from build123d import *

# Parameters (mm, degrees)
PAD_DEPTH            = 6.5
POCKET_DEPTH         = 6
SKETCH002_R          = 13.5
POCKET001_DEPTH      = 1
SKETCH003_W          = 6.45
SKETCH003_H          = 6.5
PAD001_DEPTH         = 3.5
POCKET002_DEPTH      = 10
SKETCH010_W          = 5
SKETCH010_H          = 6.5
PAD002_DEPTH         = 3.5
POCKET005_DEPTH      = 10
SKETCH015_R          = 2.2
SKETCH015_R_2        = 1.025
PAD003_DEPTH         = 2
POCKET009_DEPTH      = 4
POCKET010_DEPTH      = 4
PAD004_DEPTH         = 4
POCKET013_DEPTH      = 13.201
POCKET013_DEPTH_BACK = 35.201
SKETCH022_R          = 0.6
POCKET014_DEPTH      = 2
SKETCH023_R          = 0.6
POCKET015_DEPTH      = 2
SKETCH024_R          = 13.5
PAD005_DEPTH         = 0.5
SKETCH025_R          = 20.45
SKETCH025_R_2        = 19.85
POCKET016_DEPTH      = 0.3
SKETCH026_R          = 1
POCKET017_DEPTH      = 5


with BuildPart() as part:
    # Sketch → Pad (new body)
    with BuildSketch(Plane.XY):
        with BuildLine():
            Line((-22.5019915649, 16), (-22.5019915649, -16))
            Line((-22.5019915649, -16), (-16.2858834578, -17.9))
            ThreePointArc((-16.2858834578, -17.9), (-0.4552796053, -24.1957169863), (15.6009615088, -18.5))
            Line((15.6009615088, -18.5), (24.5395016581, -17.45))
            Line((24.5395016581, 17.45), (24.5395016581, -17.45))
            Line((15.6009615088, 18.5), (24.5395016581, 17.45))
            ThreePointArc((15.6009615088, 18.5), (-0.4552796053, 24.1957169863), (-16.2858834578, 17.9))
            Line((-22.5019915649, 16), (-16.2858834578, 17.9))
        make_face()
    extrude(amount=PAD_DEPTH)

    # Sketch001 → Pocket (cut)
    with BuildSketch(Plane.XY):
        with BuildLine():
            Line((-14.8539557021, 16.9), (-21.2122180433, 15.55))
            Line((-21.2122180433, 15.55), (-21.2122180433, -15.55))
            Line((-21.2122180433, -15.55), (-14.8539557021, -16.9))
            ThreePointArc((-14.8539557021, -16.9), (-0.0760301383, -22.4998715423), (14.739402973, -17))
            Line((14.739402973, -17), (23.6191552218, -16.4))
            Line((23.6191552218, 16.4), (23.6191552218, -16.4))
            Line((14.739402973, 17), (23.6191552218, 16.4))
            ThreePointArc((14.739402973, 17), (-0.0760301383, 22.4998715423), (-14.8539557021, 16.9))
        make_face()
    extrude(amount=POCKET_DEPTH, mode=Mode.SUBTRACT)

    # Sketch002 (on Face19 of Pocket) → Pocket001 (cut)
    with BuildSketch(Plane(origin=(0, 0, 6), x_dir=(1, 0, 0), z_dir=(0, 0, -1))):
        Circle(SKETCH002_R)
    extrude(amount=-POCKET001_DEPTH, mode=Mode.SUBTRACT)

    # Sketch003 (on Face7 of Pad) → Pad001 (join)
    with BuildSketch(Plane.YZ.offset(24.5395016581)):
        with Locations((-14.225, 3.25)):
            Rectangle(SKETCH003_W, SKETCH003_H)
        with Locations((14.225, 3.25)):
            Rectangle(SKETCH003_W, SKETCH003_H)
    extrude(amount=PAD001_DEPTH)

    # Sketch006 (on Face22 of Pad001) → Pocket002 (cut)
    with BuildSketch(Plane.XY.offset(6.5)):
        with BuildLine():
            ThreePointArc((24.5395016581, 17.45), (26.1592830786, 16.2095505764), (28.0395016581, 15.4176006311))
            Line((28.0395016581, 17.45), (28.0395016581, 15.4176006311))
            Line((28.0395016581, 17.45), (24.5395016581, 17.45))
        make_face()
        with BuildLine():
            ThreePointArc((28.0395016581, -15.4176006311), (26.1592830786, -16.2095505765), (24.5395016581, -17.4500000001))
            Line((28.0395016581, -17.45), (24.5395016581, -17.4500000001))
            Line((28.0395016581, -15.4176006311), (28.0395016581, -17.45))
        make_face()
    extrude(amount=-POCKET002_DEPTH, mode=Mode.SUBTRACT)

    # Sketch010 (on Face3 of Pad) → Pad002 (join)
    with BuildSketch(Plane(origin=(-22.5019915649, 0, 0), x_dir=(0, -1, 0), z_dir=(-1, 0, 0))):
        with Locations((-13.5, 3.25)):
            Rectangle(SKETCH010_W, SKETCH010_H)
        with Locations((13.5, 3.25)):
            Rectangle(SKETCH010_W, SKETCH010_H)
    extrude(amount=PAD002_DEPTH)

    # Sketch011 (on Face28 of Pad002) → Pocket005 (cut)
    with BuildSketch(Plane.XY.offset(6.5)):
        Polygon((-26.0019915649, 16), (-22.5019915649, 16), (-26.0019915649, 14.5), align=None)
        Polygon((-22.5019915649, -16), (-26.0019915649, -14.5), (-26.0019915649, -16), align=None)
    extrude(amount=-POCKET005_DEPTH, mode=Mode.SUBTRACT)

    # Sketch015 (on Face19 of Pocket) → Pad003 (join)
    with BuildSketch(Plane(origin=(0, 0, 6), x_dir=(1, 0, 0), z_dir=(0, 0, -1))):
        with Locations((-18.42, 13.32)):
            Circle(SKETCH015_R)
        with Locations((-18.42, 13.32)):
            Circle(SKETCH015_R_2, mode=Mode.SUBTRACT)
        with Locations((7.27, 18.56)):
            Circle(SKETCH015_R)
        with Locations((7.27, 18.56)):
            Circle(SKETCH015_R_2, mode=Mode.SUBTRACT)
        with Locations((5.37, -19.79)):
            Circle(SKETCH015_R)
        with Locations((5.37, -19.79)):
            Circle(SKETCH015_R_2, mode=Mode.SUBTRACT)
        with Locations((-18.42, -13.32)):
            Circle(SKETCH015_R)
        with Locations((-18.42, -13.32)):
            Circle(SKETCH015_R_2, mode=Mode.SUBTRACT)
    extrude(amount=PAD003_DEPTH)

    # Sketch016 (on Face4 of Pocket) → Pocket009 (cut)
    with BuildSketch(Plane(origin=(0, 0, 0), x_dir=(1, 0, 0), z_dir=(0, 0, -1))):
        with BuildLine():
            Line((-4.9992330338, 23.6779996848), (-5.0007669662, 21.9372361465))
            ThreePointArc((5.0007669662, 21.9372361465), (0, 22.5), (-5.0007669662, 21.9372361465))
            Line((5.0007669662, 23.6776757675), (5.0007669662, 21.9372361465))
            ThreePointArc((5.0007669662, 23.6776757675), (0.00078388, 24.1999999873), (-4.9992330338, 23.6779996848))
        make_face()
    extrude(amount=-POCKET009_DEPTH, mode=Mode.SUBTRACT)

    # Sketch017 (on Face4 of Pocket) → Pocket010 (cut)
    with BuildSketch(Plane(origin=(0, 0, 0), x_dir=(1, 0, 0), z_dir=(0, 0, -1))):
        with BuildLine():
            ThreePointArc((-3.2541322314, -22.2634369184), (0, -22.5), (3.2541322314, -22.2634369184))
            Line((3.2541322314, -22.2634369184), (3.5, -23.9455632634))
            ThreePointArc((-3.5, -23.9455632634), (0, -24.2), (3.5, -23.9455632634))
            Line((-3.2541322314, -22.2634369184), (-3.5, -23.9455632634))
        make_face()
        with BuildLine():
            ThreePointArc((-13.9498796389, -17.6536358312), (-11.25, -19.4855715851), (-8.3135572795, -20.9077680626))
            Line((-8.3135572795, -20.9077680626), (-8.9416927184, -22.487466094))
            ThreePointArc((-15.0038705449, -18.987466094), (-12.1, -20.9578147716), (-8.9416927184, -22.487466094))
            Line((-13.9498796389, -17.6536358312), (-15.0038705449, -18.987466094))
        make_face()
        with BuildLine():
            ThreePointArc((8.3135572795, -20.9077680626), (11.25, -19.4855715851), (13.9498796389, -17.6536358312))
            Line((13.9498796389, -17.6536358312), (15.0038705449, -18.987466094))
            ThreePointArc((8.9416927184, -22.487466094), (12.1, -20.9578147716), (15.0038705449, -18.987466094))
            Line((8.3135572795, -20.9077680626), (8.9416927184, -22.487466094))
        make_face()
    extrude(amount=-POCKET010_DEPTH, mode=Mode.SUBTRACT)

    # Sketch018 (on Face8 of Pocket005) → Pad004 (join)
    with BuildSketch(Plane(origin=(0, 0, 0), x_dir=(1, 0, 0), z_dir=(0, 0, -1))):
        Polygon((-26.0019915649, 14.5), (-26.0019915649, 11), (-22.5019915649, 11), (-22.5019915649, 16), align=None)
        Polygon((-26.0019915649, -11), (-22.5019915649, -11), (-22.5019915649, -16), (-26.0019915649, -14.5), align=None)
        with BuildLine():
            Line((24.5395016581, 17.4500000001), (24.5395016581, 11))
            Line((28.0395016581, 11), (24.5395016581, 11))
            Line((28.0395016581, 15.4176006311), (28.0395016581, 11))
            ThreePointArc((24.5395016581, 17.4500000001), (26.1592830786, 16.2095505765), (28.0395016581, 15.4176006311))
        make_face()
        with BuildLine():
            Line((24.5395016581, -11), (24.5395016581, -17.45))
            ThreePointArc((28.0395016581, -15.4176006311), (26.1592830786, -16.2095505764), (24.5395016581, -17.45))
            Line((28.0395016581, -11), (28.0395016581, -15.4176006311))
            Line((24.5395016581, -11), (28.0395016581, -11))
        make_face()
    extrude(amount=PAD004_DEPTH)

    # Sketch021 (on Face50 of Pad004) → Pocket013 (cut, two sides)
    with BuildSketch(Plane(origin=(0, -11, 0), x_dir=(-1, 0, 0), z_dir=(0, 1, 0))) as pocket013_sk:
        with BuildLine():
            Line((-24.5395016581, -4), (-24.5395016581, -2))
            ThreePointArc((-26.5395016581, -4), (-25.1252880957, -3.4142135624), (-24.5395016581, -2))
            Line((-24.5395016581, -4), (-26.5395016581, -4))
        make_face()
        with BuildLine():
            Line((22.5019915649, -4), (22.5019915649, -2))
            ThreePointArc((22.5019915649, -2), (23.0877780026, -3.4142135624), (24.5019915649, -4))
            Line((22.5019915649, -4), (24.5019915649, -4))
        make_face()
        with BuildLine():
            Line((-28.0395016581, 0), (-28.0395016581, 6.5))
            Line((-28.0395016581, 6.5), (-24.5395016581, 6.5))
            ThreePointArc((-24.5395016581, 6.5), (-27.1088837932, 3.6912057651), (-28.0395016581, 0))
        make_face()
        with BuildLine():
            Line((26.0019915649, 6.5), (26.0019915649, 0))
            ThreePointArc((26.0019915649, 0), (25.0713737, 3.6912057651), (22.5019915649, 6.5))
            Line((26.0019915649, 6.5), (22.5019915649, 6.5))
        make_face()
    extrude(amount=-POCKET013_DEPTH, mode=Mode.SUBTRACT)
    extrude(pocket013_sk.sketch, amount=POCKET013_DEPTH_BACK, mode=Mode.SUBTRACT)

    # Sketch022 (on Face66 of Pocket013) → Pocket014 (cut)
    with BuildSketch(Plane.XZ.offset(-11)):
        with Locations((-24.7019915649, -2.7)):
            Circle(SKETCH022_R)
        with Locations((26.7395016581, -2.7)):
            Circle(SKETCH022_R)
    extrude(amount=-POCKET014_DEPTH, mode=Mode.SUBTRACT)

    # Sketch023 (on Face49 of Pocket014) → Pocket015 (cut)
    with BuildSketch(Plane(origin=(0, -11, 0), x_dir=(-1, 0, 0), z_dir=(0, 1, 0))):
        with Locations((-26.7395016581, -2.7)):
            Circle(SKETCH023_R)
        with Locations((24.7019915649, -2.7)):
            Circle(SKETCH023_R)
    extrude(amount=-POCKET015_DEPTH, mode=Mode.SUBTRACT)

    # Sketch024 (on Face16 of Pocket015) → Pad005 (join)
    with BuildSketch(Plane.XY.offset(6.5)):
        with BuildLine():
            ThreePointArc((-22.5019915649, -8.9050758341), (24.2, 0), (-22.5019915649, 8.9050758341))
            Line((-22.5019915649, 8.9050758341), (-22.5019915649, -8.9050758341))
        make_face()
        Circle(SKETCH024_R, mode=Mode.SUBTRACT)
    extrude(amount=PAD005_DEPTH)

    # Sketch025 (on Face42 of Pad005) → Pocket016 (cut)
    with BuildSketch(Plane.XY.offset(7)):
        Circle(SKETCH025_R)
        Circle(SKETCH025_R_2, mode=Mode.SUBTRACT)
    extrude(amount=-POCKET016_DEPTH, mode=Mode.SUBTRACT)

    # Sketch026 (on DatumPlane) → Pocket017 (cut)
    with BuildSketch(Plane.XZ.offset(25)):
        with Locations((-6.5, 4.8)):
            Circle(SKETCH026_R)
    extrude(amount=-POCKET017_DEPTH, mode=Mode.SUBTRACT)


solid = part.part
Source: CAD feature listing. Evaluate the final solid. Frame: model axes, mm. A direction names the side the tool comes from. Give positions to 0.01 mm unless a question says otherwise; leave off trailing zeros. Order: outer loops, then holes, each group sorted by start corner. A loop starts at its lowest first (then second) coordinate and runs counter-clockwise, first axis right, second up. Notation, with made-up numbers: (-15, 43.25) -> (24, 43.25) arc R23 ccw to (24, 79.25) -> close; hole circle Ø9 at (-27.75, 11.25). An arc over 180 degrees is marked (long way). Write item = value, one per line.
Item 1: Section query B-B (x = 0). Output: boundary loops of the cut face in (y, z).
Check result:
outline = (-24.2, 4) -> (-22.5, 4) -> (-22.5, 6) -> (-13.5, 6) -> (-13.5, 7) -> (-19.85, 7) -> (-19.85, 6.7) -> (-20.45, 6.7) -> (-20.45, 7) -> (-24.2, 7) -> close; (13.5, 6) -> (22.5, 6) -> (22.5, 4) -> (24.2, 4) -> (24.2, 7) -> (20.45, 7) -> (20.45, 6.7) -> (19.85, 6.7) -> (19.85, 7) -> (13.5, 7) -> close
Item 2: Mould query, pull axis Z, two halves, no side actions, for faces 1 (the face through (-25, -13, -3)), 2 (the face through (26, 11, 1)), 3 (the face through (24.1, -4, 6.5)). Classes: +Z half, -Z half, draft (parallel to the pull), parting line (faces both ways), or undercut.
Check result:
face_1 = undercut
face_2 = draft
face_3 = +Z half
Item 3: Contact query for flat-ended pins moving along their axis: pin 1 (1 mm diameter, centred on x = 26.5, z = -2.5, fed in from -Y); pin 2 (0.6 mm diameter, centred on x = 0, y = 23.5, fed in from -Z); pin 3 (19.5 mm diameter, centred on x = -14.5, y = -10.5, fed in from -Z). Output: stop coordinate, or through.
Check result:
pin_1 = -16.3
pin_2 = 4
pin_3 = -3.98
Item 4: Ray query, probe 1 along X at (y, z) = (-13.32, 4.6) (3 decimals); probe 2 along Y at (x, z) = (-18, 5) (3 decimals); probe 3 along X at (y, z) = (0, 6.55). Return the intervals inside material, ascending.
Check result:
probe_1 = -24.498 to -21.212, -20.62 to -19.445, -17.395 to -16.22, 23.619 to 26.535
probe_2 = -17.376 to -16.232, -15.48 to -14.255, -12.385 to -11.16, 11.16 to 12.385, 14.255 to 15.48, 16.232 to 17.376
probe_3 = -22.5 to -13.5, 13.5 to 24.2
Item 5: Set-up query: faces 4 (the face through (-24.23, 15.26, 0.16)), 5 (the face through (-14.47, 18.31, 1.97)), 6 (the face through (-22.502, 13, -1)), 7 (the face through (-19.444, -13.365, 5.014)), 8 (the face through (-24.1, -12, -2.7)). Return all of +Z, -Z, +X, -X, +Y, -Y with unobstructed straight access to the full face (end or side cutting, diameter ignored); none if empty.
Check result:
face_4 = +Z, -Z, -X, +Y
face_5 = -Z, +Y
face_6 = -Z, +Y, -Y
face_7 = -Z
face_8 = none
Item 6: Section query C-C (z = 4.8). State how many separate pieces and enclosed holes the cut face has, then the cut area to 3 significant figures.
Check result:
separate_pieces = 4
enclosed_holes = 4
area = 305 mm²
Item 7: Section query A-A (y = 0). Output: boundary loops of the cut face in (x, z), then the cut area to 3 significant figures.
Check result:
outline = (-22.5, 0) -> (-21.21, 0) -> (-21.21, 6) -> (-13.5, 6) -> (-13.5, 7) -> (-19.85, 7) -> (-19.85, 6.7) -> (-20.45, 6.7) -> (-20.45, 7) -> (-22.5, 7) -> close; (13.5, 6) -> (23.62, 6) -> (23.62, 0) -> (24.54, 0) -> (24.54, 6.5) -> (24.2, 6.5) -> (24.2, 7) -> (20.45, 7) -> (20.45, 6.7) -> (19.85, 6.7) -> (19.85, 7) -> (13.5, 7) -> close
area = 32.8 mm²
